Input: part model. Units: mm. Frame: model coordinates. A direction names the side the tool comes from. Coordinates: 2 decimals unless noted, no trailing zeros. Write each loop counter-clockwise with the first axis right and the second up, starting at its lowest first coordinate (ties: lowest second). Pieces come first, ordered by that corner, then holes. Notation, with made-up numbers: M -33,58 L 18,58 A4 ccw 18,64 Z; hole C -24,45.5 d11. An arc over 180 degrees is marked long. Write each question's results on one line, items separated by ' | '. Start each with the question number.
1. Pull-direction query (Z, two-part tool) for faces 1 (the flat face through (-31.75, 1, 57)), 2 (the cylindrical face through (-38.645, -0.827, 73.157)), 3 (the flat face through (0, 0, 0)); classes: +Z half, -Z half, draft (parallel to the pull), parting line (faces both ways), or undercut.
2. Section query A-A, the plane y = 2.5. Count the separate pieces of the cut face and the enclosed holes in it, and give its area (3 significant figures).
3. Set-up query: faces 4 (the flat face through (0, 1, 44.45)), 5 (the conical face through (15.06, -28.95, 21.7)). Return all of +Z, -Z, +X, -X, +Y, -Y with unobstructed straight access to the full face (end or side cutting, diameter ignored); none if empty.
4. First-contact query: pin 1 (1.5 mm diameter, centred on y = 11.5, z = 12, fed in from -X); pin 2 (1.5 mm diameter, centred on x = 13.5, z = 30, fed in from -Y); pin 3 (2 mm diameter, centred on x = -8.5, y = -10.5, fed in from +Z); pin 4 (20.5 mm diameter, centred on y = 0, z = 66.86, fed in from -X). Flat tips, straight axial feed; report the tip coordinate or a pass-through.
5. Ray query, probe 1 along Z at (x, y) = (-23, -8.5); probe 2 along X at (y, z) = (-29, 60); probe 3 along X at (y, z) = (-14, 66). Return the intervals inside material, ascending.
6. Section query C-C, the plane z = 47. Output: boundary loops of the cut face in (x, y), and give its area (3 significant figures).
7. Section query B-B, the plane x = 0. Output: boundary loops of the cut face in (y, z), and give its area (3 significant figures).
8. Section query D-D, the plane z = 29. Output: boundary loops of the cut face in (x, y).
```python
from build123d import *

# Parameters (mm, degrees)
F0_R     = 25.4
F2_R     = 50.8
F5_DEPTH = 31.75
F7_R     = 6.35
F8_DEPTH = 127


# Not quite as in the source:
# - a feature names something its author has since deleted; it is built from what else it names


with BuildPart() as f3:
    # F0 (on Top) → F3 section 0
    with BuildSketch(Plane.XY):
        Circle(F0_R)
    # F2 (on offset) → F3 section 1
    with BuildSketch(Plane.XY.offset(76.2)):
        Circle(F2_R)
    loft()

    # F4 (on face) → F5 (cut)
    with BuildSketch(Plane.XY.offset(76.2)):
        with BuildLine():
            Line((31.75, -39.6557372898), (31.75, 39.6557372898))
            ThreePointArc((31.75, 39.6557372898), (0, 50.8), (-31.75, 39.6557372898))
            Line((-31.75, 39.6557372898), (-31.75, -39.6557372898))
            ThreePointArc((-31.75, -39.6557372898), (0, -50.8), (31.75, -39.6557372898))
        make_face()
    extrude(amount=-F5_DEPTH, mode=Mode.SUBTRACT)

    # F7 (on offset) → F8 (cut)
    with BuildSketch(Plane.YZ.offset(50.8)):
        with Locations((0, 66.8615028262)):
            Circle(F7_R)
    extrude(amount=-F8_DEPTH, mode=Mode.SUBTRACT)


solid = f3.part
```
Answer:
1) face 1: draft | face 2: undercut | face 3: -Z half
2) separate pieces: 3 | enclosed holes: 0 | area: 3,410 mm^2
3) face 4: +Z, +Y, -Y | face 5: -Z
4) pin 1: x = -27.47 | pin 2: y = -33.13 | pin 3: z = 44.45 | pin 4: x = -50.8
5) probe 1: 0 to 44.45 | probe 2: -34.93 to -31.75, 31.75 to 34.93 | probe 3: -45.29 to -31.75, 31.75 to 45.29
6) outline: M -31.75,-26.05 L -31.75,26.05 A41.07 ccw Z; M 31.75,-26.05 A41.07 ccw 31.75,26.05 Z | area: 663 mm^2
7) outline: M -40.22,44.45 L -25.4,0 L 25.4,0 L 40.22,44.45 Z | area: 2,920 mm^2
8) outline: C 0,0 d70.13
